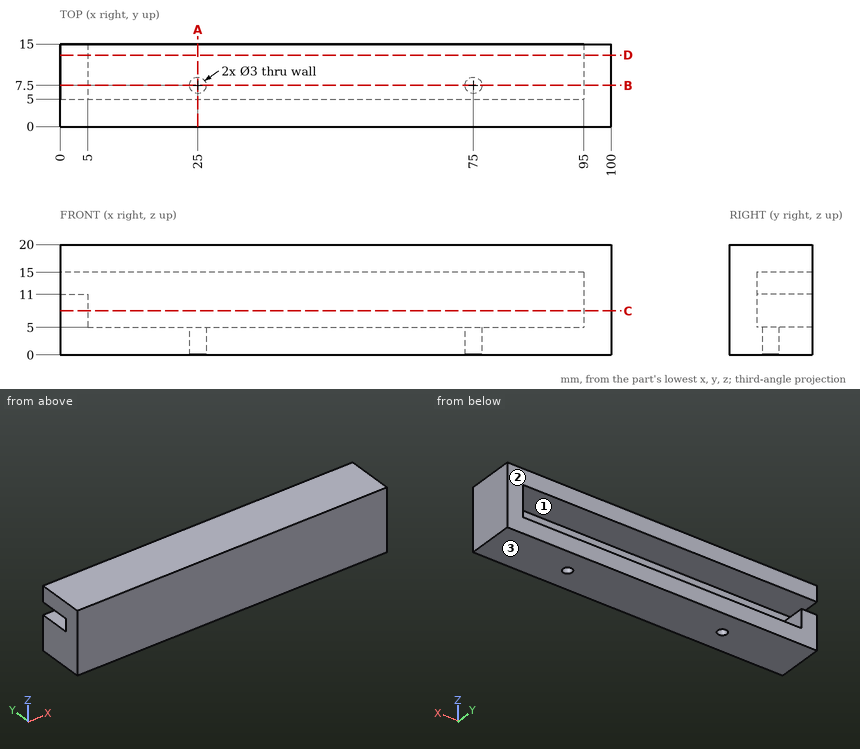
For this review, use the dimensioned drawing (mm, ordinates from the lowest corner) and the shaded views. Round coordinates to 2 decimals unless told otherwise and drop trailing zeros. Write each loop counter-clockwise with the first axis right and the second up, starting at its lowest first coordinate (ties: lowest second). Pieces come first, ordered by that corner, then holes. Notation, with made-up numbers: (89, 8) - (124, 8) arc R21 ccw to (124, 21) - close; hole circle Ø11 at (27, 11). An arc over 180 degrees is marked (long way). One line per item, written item: value. Start each with the question number.
1. To check wall thickness, follow L1, parallel to Z at x = 69, y = 9; L2, parallel to Y at x = 75, z = 3.1; L3, parallel to X at y = 10.5, z = 10.5. State the ranges of each line that lie inside material, in increasing order. Write a range as from..to.
2. Consider section B-B on y = 7.5. Write out the cut boundary in (x, z).
3. Consider section A-A on x = 25. Write out the cut boundary in (y, z), and give its area (3 significant figures).
4. Consider section D-D on y = 13. Write out the cut boundary in (x, z), and give its area (3 significant figures).
5. The part is to be moulded in two halves that separate along Z. For the marked faces 1, 2 and 3, say which applies: released by +Z, released by -Z, zero draft, split by the parting line, or undercut.
6. Consider section C-C on z = 8. Write out the cut boundary in (x, y), and give its area (3 significant figures).
7. Clearance check with a flat-ended pin moving along its axis: P1, Ø5, axis at x = 56.5, z = 10, coming from the +Y side. State where the tip first meets the part, or that it passes through.
Checks:
1. L1: z = 0..5, 15..20
1. L2: y = 0..6, 9..15
1. L3: x = 0..5, 95..100
2. outline: (0, 0) - (23.5, 0) - (23.5, 5) - (5, 5) - (5, 11) - (0, 11) - close; (0, 15) - (95, 15) - (95, 5) - (76.5, 5) - (76.5, 0) - (100, 0) - (100, 20) - (0, 20) - close; (26.5, 0) - (73.5, 0) - (73.5, 5) - (26.5, 5) - close
3. outline: (0, 0) - (6, 0) - (6, 5) - (5, 5) - (5, 15) - (15, 15) - (15, 20) - (0, 20) - close; (9, 0) - (15, 0) - (15, 5) - (9, 5) - close
3. area: 185 mm^2
4. outline: (0, 0) - (100, 0) - (100, 20) - (0, 20) - (0, 15) - (95, 15) - (95, 5) - (5, 5) - (5, 11) - (0, 11) - close
4. area: 1,080 mm^2
5. face 1: undercut
5. face 2: zero draft
5. face 3: released by -Z
6. outline: (0, 0) - (100, 0) - (100, 15) - (95, 15) - (95, 5) - (5, 5) - (5, 15) - (0, 15) - close
6. area: 600 mm^2
7. P1: stops at y = 5
